from build123d import *

# Parameters (mm, degrees)
F0_R     = 21.5
F1_DEPTH = 40
F2_R     = 10
F5_DEPTH = 12
F3_R     = 10
F6_DEPTH = 12
F4_R     = 10
F7_DEPTH = 12


# Not quite as in the source:
# - a feature names something its author has since deleted; it is built from what else it names


with BuildPart() as f1:
    # F0 (on Top) → F1 (new body)
    with BuildSketch(Plane.XY):
        with BuildLine():
            Line((7.6794919243, 53.3012701892), (-2.9591014593, 34.8746859277))
            ThreePointArc((-2.9591014593, 34.8746859277), (-17.5, 30.3108891325), (-28.7228132327, 20))
            Line((-28.7228132327, 20), (-50, 20))
            Line((-50, 20), (-50, -20))
            Line((-50, -20), (-28.7228132327, -20))
            ThreePointArc((-28.7228132327, -20), (-17.5, -30.3108891325), (-2.9591014593, -34.8746859277))
            Line((-2.9591014593, -34.8746859277), (7.6794919243, -53.3012701892))
            Line((7.6794919243, -53.3012701892), (42.3205080757, -33.3012701892))
            Line((42.3205080757, -33.3012701892), (31.681914692, -14.8746859277))
            ThreePointArc((31.681914692, -14.8746859277), (35, 0), (31.681914692, 14.8746859277))
            Line((31.681914692, 14.8746859277), (42.3205080757, 33.3012701892))
            Line((42.3205080757, 33.3012701892), (7.6794919243, 53.3012701892))
        make_face()
        Circle(F0_R, mode=Mode.SUBTRACT)
    extrude(amount=-F1_DEPTH)

    # F2 (on face) → F5 (cut)
    with BuildSketch(Plane(origin=(-50, 0, 0), x_dir=(0, -1, 0), z_dir=(-1, 0, 0))):
        with Locations((0, -20)):
            Circle(F2_R)
    extrude(amount=-F5_DEPTH, mode=Mode.SUBTRACT)

    # F3 (on face) → F6 (cut)
    with BuildSketch(Plane(origin=(25, -43.3012701892, 0), x_dir=(0.8660254038, 0.5, 0), z_dir=(0.5, -0.8660254038, 0))):
        with Locations((0, -20)):
            Circle(F3_R)
    extrude(amount=-F6_DEPTH, mode=Mode.SUBTRACT)

    # F4 (on face) → F7 (cut)
    with BuildSketch(Plane(origin=(25, 43.3012701892, 0), x_dir=(-0.8660254038, 0.5, 0), z_dir=(0.5, 0.8660254038, 0))):
        with Locations((0, -20)):
            Circle(F4_R)
    extrude(amount=-F7_DEPTH, mode=Mode.SUBTRACT)


solid = f1.part
Here's how the part is built. I have some questions about the finished solid (model axes, mm). A direction names the side the tool comes from. Coordinates: 2 decimals unless noted, no trailing zeros. Loops run counter-clockwise (first coordinate to the right, second up) from the corner with the lowest first, then second, coordinate; pieces in that order, holes last.
1. For P1, Ø12, axis at y = 0, z = -20, coming from the +X side; P2, Ø4, axis at x = -22, z = -16.5, coming from the +Y side; P3, Ø23.5, axis at x = -40, z = -14, coming from the +Y side, each with a flat end and sliding along its axis, tell me the tip position at first contact or that it passes through.
2. Imagine slicing it at B-B, the plane x = 0. Please give me the cut outline in (y, z), and give its area (3 significant figures).
3. I need wall thicknesses on L1, parallel to Z at x = -47, y = 0; L2, parallel to Y at x = -42.5, z = -36.5; L3, parallel to X at y = 8, z = -10. Which ranges of each line are inside material? Lowest first, please.
4. Imagine slicing it at D-D, the plane x = -13. Please give me the cut outline in (y, z).
5. If we mould it in two halves opening along X, with no side actions, what happens to faces 6 (the flat face through (19.12, 32.84, -19.86)), 7 (the cylindrical face through (17.386, 40.866, -11.568)), 8 (the flat face through (-38, 0, -20)), 9 (the flat face through (37.076, -24.217, -19.72))? For each: pulls with the +X half, pulls with the -X half, needs draft (parallel to the pull), parting line crosses it, or undercut.
6. Imagine slicing it at C-C, the plane z = -5. Please give me the cut outline in (x, y).
7. For faces 1 (the flat face through (-39, 20, -20)), 2 (the cylindrical face through (-44.084, 1.302, -10.085)), 3 (the flat face through (36.927, 23.959, -19.72)), 4 (the flat face through (18.88, -32.98, -19.86)), 5 (the flat face through (2.286, -43.959, -19.72)), which set-ups out of +Z, -Z, +X, -X, +Y, -Y let a thin tool reach every point of the face, with its end or its side?
8. Imagine slicing it at A-A, the plane y = 0. Please give me the cut outline in (x, z).
Taken from the geometry:
1. P1: stops at x = 35
1. P2: stops at y = 28.72
1. P3: stops at y = 20.66
2. outline: (-40, -40) - (-21.5, -40) - (-21.5, 0) - (-40, 0) - close; (21.5, -40) - (40, -40) - (40, 0) - (21.5, 0) - close
2. area: 1,480 mm2
3. L1: z = -40 to -30, -10 to 0
3. L2: y = -20 to 20
3. L3: x = -50 to -19.96, 19.96 to 34.07
4. outline: (-32.5, -40) - (-17.12, -40) - (-17.12, 0) - (-32.5, 0) - close; (17.12, -40) - (32.5, -40) - (32.5, 0) - (17.12, 0) - close
5. face 6: undercut
5. face 7: undercut
5. face 8: pulls with the -X half
5. face 9: pulls with the +X half
6. outline: (-50, -20) - (-28.72, -20) arc R35 ccw to (-2.96, -34.87) - (7.68, -53.3) - (42.32, -33.3) - (31.68, -14.87) arc R35 ccw to (31.68, 14.87) - (42.32, 33.3) - (7.68, 53.3) - (-2.96, 34.87) arc R35 ccw to (-28.72, 20) - (-50, 20) - close; hole circle Ø43 at (0, 0)
7. face 1: +Z, -Z, -X, +Y
7. face 2: -X
7. face 3: +Z, -Z, +X
7. face 4: none
7. face 5: +Z, -Z, -X, -Y
8. outline: (-50, -40) - (-21.5, -40) - (-21.5, 0) - (-50, 0) - (-50, -10) - (-38, -10) - (-38, -30) - (-50, -30) - close; (21.5, -40) - (35, -40) - (35, 0) - (21.5, 0) - close
